from build123d import *

# Parameters (mm, degrees)
SKETCH_R  = 1.6
PAD_DEPTH = 1.6


with BuildPart() as part:
    # Sketch → Pad (new body)
    with BuildSketch(Plane.XY):
        with BuildLine():
            Line((-10.87834, 42.048496), (21.88766, 42.048496))
            Line((21.88766, 42.048496), (24.42766, 39.508496))
            Line((24.42766, 39.508496), (25.96766, 39.508496))
            ThreePointArc((26.96766, 38.508496), (26.674767, 39.215603), (25.96766, 39.508496))
            Line((26.96766, 38.508496), (26.96766, -25.531504))
            ThreePointArc((25.96766, -26.531504), (26.674767, -26.238611), (26.96766, -25.531504))
            Line((25.96766, -26.531504), (-25.37234, -26.531504))
            ThreePointArc((-26.37234, -25.531504), (-26.079447, -26.238611), (-25.37234, -26.531504))
            Line((-26.37234, -25.531504), (-26.37234, 37.984496))
            Line((-26.37234, 37.984496), (-24.84834, 39.508496))
            Line((-24.84834, 39.508496), (-13.41834, 39.508496))
            Line((-13.41834, 39.508496), (-10.87834, 42.048496))
        make_face()
        with Locations((24.42766, -12.561504)):
            Circle(SKETCH_R, mode=Mode.SUBTRACT)
        with Locations((-23.83234, -11.291504)):
            Circle(SKETCH_R, mode=Mode.SUBTRACT)
        with Locations((-8.59234, 39.508496)):
            Circle(SKETCH_R, mode=Mode.SUBTRACT)
        with Locations((19.34766, 39.508496)):
            Circle(SKETCH_R, mode=Mode.SUBTRACT)
    extrude(amount=PAD_DEPTH)


solid = part.part
CAD build for the part. Positions are in the model's coordinates, mm. A direction names the side the tool comes from. Round coordinates to 2 decimals unless told otherwise and drop trailing zeros. Write each loop counter-clockwise with the first axis right and the second up, starting at its lowest first coordinate (ties: lowest second). Pieces come first, ordered by that corner, then holes.
(1) Mould opens along X. For faces 1 (the face through (-8.801, 41.095, 0.789)), 2 (the face through (-12.166, 40.761, 0.789)), 3 (the face through (-19, 39.508, 1)), 4 (the face through (26.968, 7, 1)) say: pulls with the +X half, pulls with the -X half, needs draft (parallel to the pull), parting line crosses it, or undercut.
(2) Probe line 1 along Y through (x, z) = (-18, 0.85); line 2 along Y through (x, z) = (20, 0.95); line 3 along Y through (x, z) = (23.5, 1.35). List the from-to ranges inside material, lowest first.
(3) Slice it at A-A, the plane x = -9. Write the cut outline in (y, z), and give its area (3 significant figures).
(4) Slice it at B-B, the plane z = 0.6. Write the cut outline in (x, y).
(5) Slice it at C-C, the plane x = -17. Write the cut outline in (y, z), and give its area (3 significant figures).
(6) Drop a flat-ended pin along its axis: P1, Ø1.9, axis at x = 19.35, y = 39.51, coming from the +Z side. Give the stop position or say it passes through.
(7) 3-axis set-ups, long thin cutter, end or side, ignore diameter. For faces 5 (the face through (1, 8, 1.6)), 6 (the face through (25, 39.508, 1)): which of +Z, -Z, +X, -X, +Y, -Y reach the whole face in a straight line?
From the geometry:
1. face 1: undercut
1. face 2: pulls with the -X half
1. face 3: needs draft
1. face 4: pulls with the +X half
2. line 1: y = -26.53 to 39.51
2. line 2: y = -26.53 to 38.05, 40.97 to 42.05
2. line 3: y = -26.53 to -13.87, -11.26 to 40.44
3. outline: (-26.53, 0) - (37.96, 0) - (37.96, 1.6) - (-26.53, 1.6) - close; (41.06, 0) - (42.05, 0) - (42.05, 1.6) - (41.06, 1.6) - close
3. area: 105 mm2
4. outline: (-26.37, -25.53) arc R1 ccw to (-25.37, -26.53) - (25.97, -26.53) arc R1 ccw to (26.97, -25.53) - (26.97, 38.51) arc R1 ccw to (25.97, 39.51) - (24.43, 39.51) - (21.89, 42.05) - (-10.88, 42.05) - (-13.42, 39.51) - (-24.85, 39.51) - (-26.37, 37.98) - close; hole circle Ø3.2 at (-23.83, -11.29); hole circle Ø3.2 at (-8.59, 39.51); hole circle Ø3.2 at (19.35, 39.51); hole circle Ø3.2 at (24.43, -12.56)
5. outline: (-26.53, 0) - (39.51, 0) - (39.51, 1.6) - (-26.53, 1.6) - close
5. area: 106 mm2
6. P1: passes through
7. face 5: +Z, +X, -X, +Y, -Y
7. face 6: +Z, -Z, +X, +Y
